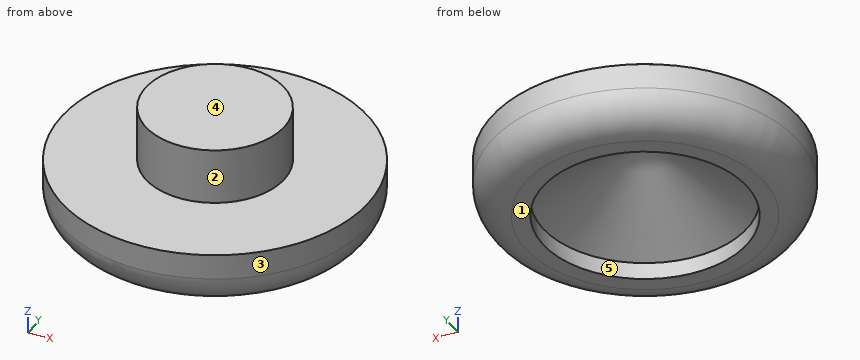
from build123d import *

# Parameters (mm, degrees)
F0_R     = 4.075
F1_DEPTH = 6.8
F0_R_2   = 9
F2_DEPTH = 3.5
F3_R     = 2
F4_D     = 12
F4_DEPTH = 1
F4_TIP   = 3.6051637142


with BuildPart() as f1:
    # F0 (on Top) → F1 (new body)
    with BuildSketch(Plane.XY):
        Circle(F0_R)
    extrude(amount=F1_DEPTH)

    # F0 (on Top) → F2 (join)
    with BuildSketch(Plane.XY):
        Circle(F0_R_2)
        Circle(F0_R, mode=Mode.SUBTRACT)
    extrude(amount=F2_DEPTH)

    # F3
    f3_edges = [f1.edges().sort_by_distance(p)[0] for p in [
        (-9, 0, 0),
    ]]
    fillet(f3_edges, radius=F3_R)

    # F4
    with Locations(Plane(origin=(0, 0, 0), x_dir=(1, 0, 0), z_dir=(0, 0, -1))):
        with Locations((0, 0)):
            Hole(F4_D / 2, depth=F4_DEPTH)
            with Locations((0, 0, -(F4_DEPTH + F4_TIP / 2))):  # 118° drill point
                Cone(0, F4_D / 2, F4_TIP, mode=Mode.SUBTRACT)


solid = f1.part
Design review of the part built by this model. Coordinates are the model's own, in mm. Face numbers are marked on the shaded views. A direction names the side the tool comes from. Give positions to 0.01 mm unless a question says otherwise; leave off trailing zeros. Order: outer loops, then holes, each group sorted by start corner. A loop starts at its lowest first (then second) coordinate and runs counter-clockwise, first axis right, second up. Notation, with made-up numbers: (86.25, 7.5) - (138.25, 7.5) arc R34 ccw to (138.25, 39.5) - close; hole circle Ø10 at (26.5, -39). An arc over 180 degrees is marked (long way). Write item = value, one per line. Start each with the question number.
Q1. We need section A-A on z = 5.5. State the section outline as (x, y) points (3 decimals).
Q2. We need section B-B on z = 3. State the section outline as (x, y) points.
Q3. Tool access review of the marked faces 1 and 2: name each direction out of +Z, -Z, +X, -X, +Y, -Y from which nothing blocks a thin tool from reaching the whole face with its end or side.
Q4. Mouldability with a two-part tool opening along X and no side actions: class the marked faces 3, 4 and 5 as released by +X, released by -X, zero draft, split by the parting line, or undercut.
Q5. To check wall thickness, follow L1, parallel to Z at x = -8, y = 3.5; L2, parallel to Y at x = 0, z = 0.35; L3, parallel to X at y = -0.5, z = 4. State the ranges of each line that lie inside material, in increasing order. Write a range as from..to.
Q6. Clearance check with flat-ended pins moving along their axes: pin 1 Ø1 at (x, z) = (3.5, 4.5) entering from +Y; pin 2 Ø1.5 at (x, z) = (6.5, 4.5) entering from -Y; pin 3 Ø1.5 at (x, z) = (-2, 5.5) entering from -Y. State where each tip first meets the part, or that it passes through.
Working result:
q1.outline = circle Ø8.15 at (0, 0)
q2.outline = circle Ø18 at (0, 0); hole circle Ø5.34 at (0, 0)
q3.face_1 = -Z, +X, -X, +Y, -Y
q3.face_2 = +Z
q4.face_3 = split by the parting line
q4.face_4 = zero draft
q4.face_5 = undercut
q5.L1 = 1..3.5
q5.L2 = -8.13..-6, 6..8.13
q5.L3 = -4.04..-0.87, 0.87..4.04
q6.pin_1 = 2.76
q6.pin_2 = through
q6.pin_3 = -3.88
